Verification items for the finished model (mm, model axes). Round coordinates to 2 decimals unless told otherwise and drop trailing zeros. Write each loop counter-clockwise with the first axis right and the second up, starting at its lowest first coordinate (ties: lowest second). Pieces come first, ordered by that corner, then holes.
from build123d import *

# Parameters (mm, degrees)
F1_DEPTH = 0.6


with BuildPart() as f1:
    # F0 (on Front) → F1 (new body)
    with BuildSketch(Plane.XZ):
        with BuildLine():
            Line((-25.485562, 71.361825), (-66.801734, 61.113477))
            Line((-66.801734, 61.113477), (-67.904737, 6.629639))
            Line((-67.904737, 6.629639), (-9.025994, -2.930532))
            Line((-9.025994, -2.930532), (-9.372429, -2.231689))
            Line((-9.372429, -2.231689), (-29.59533, 38.562823))
            ThreePointArc((-29.59533, 38.562823), (-31.539924, 42.710382), (-28.384709, 39.389492))
            Line((-28.384709, 39.389492), (-18.222952, 31.336777))
            Line((-18.222952, 31.336777), (-10.314779, 43.521821))
            Line((-10.314779, 43.521821), (-25.485562, 71.361825))
        make_face()
        Polygon((-9.025994, -2.930532), (-67.904737, 6.629639), (-67.923154, 5.719927), (-8.346913, -4.300405), align=None)
        Polygon((-8.346913, -4.300405), (-67.923154, 5.719927), (-67.94157, 4.810214), (-7.505301, -5.99814), align=None)
        Polygon((-7.505301, -5.99814), (-67.94157, 4.810214), (-67.197253, 3.322065), (-7.505301, -6.950844), align=None)
        Polygon((-7.505301, -6.950844), (-67.197253, 3.322065), (-66.535123, 1.998238), (-7.505301, -8.160719), align=None)
        Polygon((-7.505301, -8.160719), (-66.535123, 1.998238), (-65.95441, 0.83719), (-7.505301, -9.583006), align=None)
        with BuildLine():
            Line((-7.505301, -9.583006), (-65.95441, 0.83719))
            Line((-65.95441, 0.83719), (-45.54529, -39.967726))
            ThreePointArc((-45.54529, -39.967726), (-44.018635, -43.524925), (-46.579982, -40.622539))
            Line((-46.579982, -40.622539), (-57.517279, -32.170705))
            Line((-57.517279, -32.170705), (-65.185875, -44.597834))
            Line((-65.185875, -44.597834), (-50.259132, -71.953654))
            Line((-50.259132, -71.953654), (-7.505301, -61.244757))
            Line((-7.505301, -61.244757), (-7.505301, -9.583006))
        make_face()
    extrude(amount=F1_DEPTH)


solid = f1.part
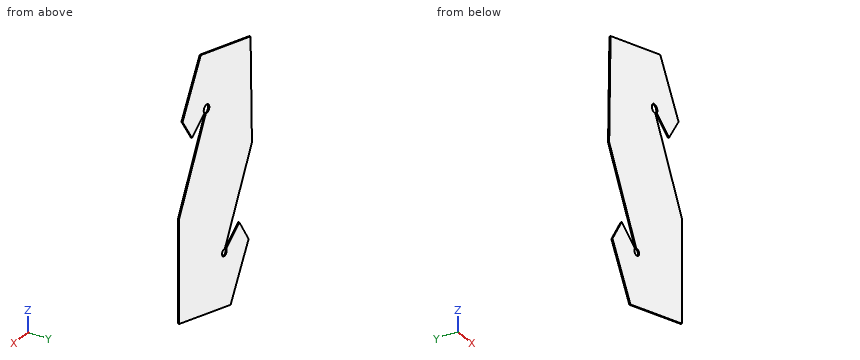
Q1. Sectioned sample at C-C (x = -15). Enter the section's corners in (y, z).
Recorded:
outline: (-0.6, -63.12) - (0, -63.12) - (0, 9.12) - (-0.6, 9.12) - close; (-0.6, 36.3) - (0, 36.3) - (0, 52.12) - (-0.6, 52.12) - close
Q2. Material ranges on line 1 along Z through (x, y) = (-19, -0.2); line 2 along Z through (x, y) = (-21, -0.1); line 3 along X through (y, z) = (-0.4, 51), recorded low to high.
Recorded:
line 1: z = -64.12 to 17.19, 31.95 to 59.46
line 2: z = -64.62 to 21.22, 33.54 to 63.13
line 3: x = -67.01 to -14.39
Q3. Sectioned sample at B-B (y = -0.3). Enter the section's corners in (x, z), plus the area to 3 significant figures.
Recorded:
outline: (-67.94, 4.81) - (-67.2, 3.32) - (-66.54, 2) - (-65.95, 0.84) - (-45.55, -39.97) arc R1.96 cw (long way) to (-46.58, -40.62) - (-57.52, -32.17) - (-65.19, -44.6) - (-50.26, -71.95) - (-7.51, -61.24) - (-7.51, -6) - (-8.35, -4.3) - (-9.03, -2.93) - (-9.37, -2.23) - (-29.6, 38.56) arc R2.32 cw (long way) to (-28.38, 39.39) - (-18.22, 31.34) - (-10.31, 43.52) - (-25.49, 71.36) - (-66.8, 61.11) - (-67.9, 6.63) - (-67.92, 5.72) - close
area: 6,650 mm2
Q4. Sectioned sample at A-A (z = 41). Enter the section's corners in (x, y), plus the area to 3 significant figures.
Recorded:
outline: (-67.21, -0.6) - (-32.54, -0.6) - (-32.54, 0) - (-67.21, 0) - close; (-27.92, -0.6) - (-11.95, -0.6) - (-11.95, 0) - (-27.92, 0) - close
area: 30.4 mm2
Q5. Sectioned sample at D-D (z = 58). Enter the section's corners in (x, y).
Recorded:
outline: (-66.86, -0.6) - (-18.2, -0.6) - (-18.2, 0) - (-66.86, 0) - close
